from build123d import *

# Parameters (mm, degrees)
F1_DEPTH = 254
F2_T     = -2.54


with BuildPart() as f1:
    # F0 (on Front) → F1 (new body)
    with BuildSketch(Plane.XZ):
        with BuildLine():
            ThreePointArc((-243.4017726194, -88.5928585449), (-220.6078758628, -99.4306883092), (-211.3480547487, -122.9099556804))
            ThreePointArc((-211.3480547487, -122.9099556804), (-220.0765697788, -145.8071744938), (-241.8322543151, -157.0836896635))
            Line((-241.8322543151, -157.0836896635), (-240.887536248, -165.8666205301))
            Line((-240.887536248, -165.8666205301), (-232.8631227599, -179.6876024772))
            ThreePointArc((-232.8631227599, -179.6876024772), (-200.2497848188, -159.2393547198), (-187.5244002098, -122.9099556804))
            ThreePointArc((-187.5244002098, -122.9099556804), (-201.2534802405, -85.358063124), (-235.9657806801, -65.5164787306))
            Line((-235.9657806801, -65.5164787306), (-243.4017726194, -88.5928585449))
        make_face()
        with BuildLine():
            ThreePointArc((-241.8322543151, -157.0836896635), (-280.1330429902, -123.6979818064), (-243.4017726194, -88.5928585449))
            Line((-243.4017726194, -88.5928585449), (-235.9657806801, -65.5164787306))
            ThreePointArc((-235.9657806801, -65.5164787306), (-303.9442391321, -124.4915476748), (-232.8631227599, -179.6876024772))
            Line((-232.8631227599, -179.6876024772), (-240.887536248, -165.8666205301))
            Line((-240.887536248, -165.8666205301), (-241.8322543151, -157.0836896635))
        make_face()
        with BuildLine():
            Line((-228.0725515097, -41.0211382589), (-235.9657806801, -65.5164787306))
            ThreePointArc((-235.9657806801, -65.5164787306), (-201.2534802405, -85.358063124), (-187.5244002098, -122.9099556804))
            ThreePointArc((-187.5244002098, -122.9099556804), (-200.2497848188, -159.2393547198), (-232.8631227599, -179.6876024772))
            Line((-232.8631227599, -179.6876024772), (-208.6762458399, -221.3462719571))
            Line((-208.6762458399, -221.3462719571), (-156.6841606223, -258.9279433801))
            Line((-156.6841606223, -258.9279433801), (-93.9011844627, -272.1134223913))
            Line((-93.9011844627, -272.1134223913), (-31.1830643044, -258.6228198834))
            Line((-31.1830643044, -258.6228198834), (20.6256671009, -220.7887835882))
            Line((20.6256671009, -220.7887835882), (52.5668094258, -165.1531620926))
            Line((52.5668094258, -165.1531620926), (59.117448986, -101.335859787))
            Line((59.117448986, -101.335859787), (39.144920691, -40.3714680019))
            Line((39.144920691, -40.3714680019), (-3.8973438724, 7.1987160788))
            Line((-3.8973438724, 7.1987160788), (-62.5669461344, 33.1493754661))
            Line((-62.5669461344, 33.1493754661), (-126.7193788673, 32.9934053975))
            Line((-126.7193788673, 32.9934053975), (-147.0301676591, 23.8912264385))
            Line((-147.0301676591, 23.8912264385), (-151.3720759465, 11.1500154879))
            Line((-151.3720759465, 11.1500154879), (-150.3917100203, 12.0439557169))
            Line((-150.3917100203, 12.0439557169), (-131.0449616301, 18.4647337066))
            Line((-131.0449616301, 18.4647337066), (-110.7592618326, 16.461374779))
            Line((-110.7592618326, 16.461374779), (-93.0421924126, 6.3802778925))
            Line((-93.0421924126, 6.3802778925), (-80.9571956273, -10.0354437172))
            Line((-80.9571956273, -10.0354437172), (-76.5938772097, -29.9473626517))
            Line((-76.5938772097, -29.9473626517), (-80.7066945537, -49.9125272331))
            Line((-80.7066945537, -49.9125272331), (-92.5845041767, -66.4787791275))
            Line((-92.5845041767, -66.4787791275), (-110.1735248884, -76.7816628826))
            Line((-110.1735248884, -76.7816628826), (-130.4324552165, -79.0397162985))
            Line((-130.4324552165, -79.0397162985), (-149.8583420607, -72.8625014256))
            Line((-149.8583420607, -72.8625014256), (-153.9562515064, -69.2190774413))
            Line((-153.9562515064, -69.2190774413), (-165.0922731069, -59.3181148339))
            Line((-165.0922731069, -59.3181148339), (-173.5001632814, -40.7485040119))
            Line((-173.5001632814, -40.7485040119), (-173.6282119898, -20.3645233703))
            Line((-173.6282119898, -20.3645233703), (-165.4542784469, -1.6907483448))
            Line((-165.4542784469, -1.6907483448), (-160.8135918091, 2.5408312775))
            Line((-160.8135918091, 2.5408312775), (-193.497810345, -3.9201981196))
            Line((-193.497810345, -3.9201981196), (-194.1558035405, -3.1681041604))
            Line((-194.1558035405, -3.1681041604), (-202.5303474039, -12.5145749574))
            Line((-202.5303474039, -12.5145749574), (-226.2911018969, -39.0329384174))
            Line((-226.2911018969, -39.0329384174), (-228.0725515097, -41.0211382589))
        make_face()
        with BuildLine():
            ThreePointArc((-202.5303474039, -12.5145749574), (-219.6834854839, -21.0493031647), (-226.2911018969, -39.0329384174))
            Line((-226.2911018969, -39.0329384174), (-202.5303474039, -12.5145749574))
        make_face()
        Polygon((-185.2621036451, 6.7577745149), (-194.1558035405, -3.1681041604), (-193.497810345, -3.9201981196), (-160.8135918091, 2.5408312775), (-151.3720759465, 11.1500154879), (-147.0301676591, 23.8912264385), align=None)
        Polygon((-220.1187830788, 26.5078867238), (-194.1558035405, -3.1681041604), (-185.2621036451, 6.7577745149), (-147.0301676591, 23.8912264385), (-140.7948214191, 42.1886792022), (-167.4157941529, 72.6167640457), (-207.0777749827, 64.7763678065), align=None)
    extrude(amount=F1_DEPTH)

    # F2
    f2_openings = [f1.faces().sort_by_distance(p)[0] for p in [
        (-102.007505, -254, -118.633515),
    ]]
    offset(amount=F2_T, openings=f2_openings, kind=Kind.INTERSECTION)


solid = f1.part
Input: part model. Units: mm. Frame: model coordinates. A direction names the side the tool comes from. Coordinates: 2 decimals unless noted, no trailing zeros. Loops run counter-clockwise (first coordinate to the right, second up) from the corner with the lowest first, then second, coordinate; pieces in that order, holes last. Notation, with made-up numbers: (38.25, -33) -> (46.25, -33) arc R32 ccw to (46.25, 0) -> close; hole circle Ø3 at (18, -9.5). An arc over 180 degrees is marked (long way). Write each question's results on one line, items separated by ' | '. Start each with the question number.
Q1. Pin query (flat end, axial travel): pin 1 (3 mm diameter, centred on y = -160, z = -234.5, fed in from -X); pin 2 (1.5 mm diameter, centred on y = -27, z = -124.5, fed in from -X); pin 3 (2 mm diameter, centred on x = -158, z = -191.5, fed in from -Y). Return the tip coordinate at first contact, or that it passes through.
Q2. Section B-B, the plane x = -22.5. Return the cut outline in (y, z).
Q3. Section C-C, the plane z = -250.5. Return the cut outline in (x, y), plus the area to 3 significant figures.
Q4. Ray query, line 1 (Z direction, x = -247, y = -29.5); line 2 (X direction, y = -16.5, z = -114); line 3 (X direction, y = -232, z = -139.5). Return the intervals inside material, ascending. Write a range as from..to.
Q5. Pull-direction query (X, two-part tool) for faces 4 (the flat face through (-207.32, -125.22, 11.88)), 5 (the flat face through (-169.24, -125.22, -50.16)), 6 (the flat face through (55.796, -125.222, -133.691)); classes: released by +X, released by -X, zero draft, split by the parting line, or undercut.
Q6. Reachability of faces 1 (the flat face through (-86.562, -125.222, -58.08)), 2 (the flat face through (-76.132, -126.51, -40.295)), 3 (the flat face through (49.27, -125.22, -71.28)) from +Z, -Z, +X, -X, +Y, -Y: full face, straight path, thin tool, end or side. Return the list, or none.
Q7. Section A-A, the plane y = -216.5. State how many separate pieces and enclosed holes the cut face has, plus the area to 3 significant figures.
Found:
1) pin 1: x = -192.55 | pin 2: x = -303.96 | pin 3: y = -2.54
2) outline: (-254, -252.28) -> (0, -252.28) -> (0, 15.43) -> (-254, 15.43) -> (-254, 12.65) -> (-2.54, 12.65) -> (-2.54, -249.14) -> (-254, -249.14) -> close
3) outline: (-168.34, -254) -> (-164.01, -254) -> (-164.01, -2.54) -> (-24.37, -2.54) -> (-24.37, -254) -> (-20.06, -254) -> (-20.06, 0) -> (-168.34, 0) -> close | area: 2,550 mm2
4) line 1: -181.12..-178.58, -159.83..-157.28, -88.54..-85.99, -67.24..-64.7 | line 2: -303.28..-300.71, -281.59..-278.97, -212.52..-209.9, 55.26..57.82 | line 3: -301.55..-298.9, -278.75..-275.88, -215.61..-212.74, 52.65..55.2
5) face 4: released by -X | face 5: undercut | face 6: released by +X
6) face 1: +Y, -Y | face 2: -Y | face 3: +Z, +X, +Y, -Y
7) separate pieces: 3 | enclosed holes: 3 | area: 4,350 mm2
